Autodesk Inventor part; units mm, degrees
ref_plane "工作平面1" through (2.5, 0, 0) normal (1, 0, 0) x (0, 1, 0)
ref_plane "工作平面3" through (0, 0, 10) normal (0, 0, 1) x (1, 0, 0)
ref_plane "工作平面4" through (0, 0, -7) normal (0, 0, 1) x (1, 0, 0)
sketch "草图1" plane through (0, 0, 0) normal (1, 0, 0) x (0, 1, 0)
  circle A0 centre (0, 0) radius 10
  dimension "d0" = 20
extrude "拉伸1" add sketch "草图1" along normal blind 80
ref_plane "工作平面1" through (2.5, 0, 0) normal (1, 0, 0) x (0, 1, 0)
sketch "草图2" plane through (2.5, 0, 0) normal (1, 0, 0) x (0, 1, 0)
  circle A0 centre (0, 0) radius 10
  line L0 (6, -2.4628) -> (-6, -2.4628)
  line L1 (-6, -2.4628) -> (-6, 2.5372)
  line L2 (-6, 2.5372) -> (6, 2.5372)
  line L3 (6, 2.5372) -> (6, -2.4628)
  line L4 (6.59, 0.0372) -> (-6.5609, 0.0372)
  point P0 (10, 0)
  point P1 (-10, 0)
  dimension "d4" = 4
  dimension "d5" = 4
  dimension "d6" = 5
extrude "拉伸2" cut sketch "草图2" along normal blind 75 contours L0 L1 L4 L3 | L4 L1 L2 L3
ref_plane "工作平面3" through (0, 0, 10) normal (0, 0, 1) x (1, 0, 0)
sketch "草图5" plane through (0, 0, 10) normal (0, 0, 1) x (1, 0, 0)
  line L0 (-2.1953, 0) -> (98.9957, 0)
  line L1 (2.5, 6) -> (2.5, -6)
  line L2 (77.5, 6) -> (77.5, -6)
  line L3 (2.5, -6) -> (2.5, 6)
  line L4 (3.5, 4) -> (76.5, 4)
  line L5 (76.5, -4) -> (3.5, -4)
  line L6 (2.5, -3) -> (2.5, -2)
  arc A0 (3.5, 4) -> (3.5, 2) centre (3.5, 3) ccw
  arc A1 (3.5, -2) -> (3.5, -4) centre (3.5, -3) ccw
  line L7 (3.5, 2) -> (76.5, 2)
  line L8 (3.5, -2) -> (76.5, -2)
  arc A2 (76.5, 2) -> (76.5, 4) centre (76.5, 3) ccw
  circle A3 centre (76.5, -3) radius 1
  point P0 (0, 0)
  point P1 (3.5, 0)
  point P2 (76.5, 0)
  dimension "d52" = 8
  dimension "d53" = 1
  dimension "d54" = 1
  dimension "d55" = 1
extrude "拉伸3" cut sketch "草图5" against normal blind 7.5 contours A0 L4 A2 L7 | A1 L8 A3 L5
ref_plane "工作平面4" through (0, 0, -7) normal (0, 0, 1) x (1, 0, 0)
sketch "草图6" plane through (0, 0, -7) normal (0, 0, 1) x (1, 0, 0)
  line L0 (0, -10) -> (0, 10)
  line L1 (80, -10) -> (80, 10)
  line L2 (0, 1) -> (80, 1)
  line L3 (80, 1) -> (80, -1)
  line L4 (80, -1) -> (0, -1)
  line L5 (0, -1) -> (0, 1)
  line L6 (-22.5072, 0) -> (150.7978, 0)
  point P0 (0, 0)
  point P1 (0, -1)
  dimension "d39" = 2
extrude "拉伸4" add sketch "草图6" against normal blind 5.5
ref_plane "工作平面5" through (2.5, -6, -2.4628) normal (0, 0, 1) x (1, 0, 0)
sketch "草图7" plane through (2.5, -6, -2.4628) normal (0, 0, 1) x (1, 0, 0)
  point P0 (-2.5, 6)
properties part number "Inner_telescope_arm"
Could you check a few things on this model? Use its own coordinates, in mm. A direction names the side the tool comes from. Give positions to 0.01 mm unless a question says otherwise; leave off trailing zeros. Order: outer loops, then holes, each group sorted by start corner. A loop starts at its lowest first (then second) coordinate and runs counter-clockwise, first axis right, second up.
Item 1: I need wall thicknesses on line 1 (Z direction, x = 74, y = 0.25); line 2 (X direction, y = 5.5, z = 0.5); line 3 (Y direction, x = 19.5, z = 6.75). Which ranges of each line are inside material? Lowest first, please.
Item 2: If we section it at C-C, the plane y = 0: Write out the boundary of the cut face in (x, z), plus the area to 4 significant figures.
Item 3: I'm going to push flat-ended pins straight in: pin 1 (2.5 mm diameter, centred on x = 37, z = -1, fed in from +Y); pin 2 (5.5 mm diameter, centred on x = 50, z = 6, fed in from -Y); pin 3 (10 mm diameter, centred on x = 61, y = -6.5, fed in from -Z); pin 4 (6 mm diameter, centred on x = 30.5, z = 4.5, fed in from -Y). Where does each tip first touch, or does it pass through?
Item 4: For faces 5 (the face through (2.5, 3, 6.2)), 6 (the face through (39, 6, 0)), 7 (the face through (39, 0, -12.5)), which set-ups out of +Z, -Z, +X, -X, +Y, -Y let a thin tool reach every point of the face, with its end or its side?
Item 5: If we section it at A-A, the plane z = 0: Write out the boundary of the cut face in (x, y), plus the area to 3 significant figures.
Item 6: If we section it at D-D, the plane z = 3.75: Write out the boundary of the cut face in (x, y).
Item 7: If we section it at B-B, the plane x = 21: Write out the boundary of the cut face in (y, z).
Item 8: If we mould it in two halves opening along X, with no side actions, what happens to faces 1 (the face through (41, -1, -11)), 2 (the face through (77.5, 3, 6.2)), 3 (the face through (0, 0, -1)), 4 (the face through (80, 0, -1))? For each: pulls with the +X half, pulls with the -X half, needs draft (parallel to the pull), parting line crosses it, or undercut.
Values:
1. line 1: z = -12.5 to -2.46, 2.54 to 10
1. line 2: x = 0 to 2.5, 77.5 to 80
1. line 3: y = -7.38 to -4, -2 to 2, 4 to 7.38
2. outline: (0, -12.5) - (80, -12.5) - (80, 10) - (0, 10) - close; hole (2.5, -2.46) - (77.5, -2.46) - (77.5, 2.54) - (2.5, 2.54) - close
2. area: 1,425 mm2
3. pin 1: stops at y = 10
3. pin 2: stops at y = -9.46
3. pin 3: stops at z = -9.89
3. pin 4: stops at y = -9.89
4. face 5: +Z
4. face 6: none
4. face 7: -Z, +X, -X, +Y, -Y
5. outline: (0, -10) - (80, -10) - (80, 10) - (0, 10) - close; hole (2.5, -6) - (77.5, -6) - (77.5, 6) - (2.5, 6) - close
5. area: 700 mm2
6. outline: (0, -9.27) - (80, -9.27) - (80, 9.27) - (0, 9.27) - close; hole (3.5, -4) - (76.5, -4) arc R1 cw to (76.5, -2) - (3.5, -2) arc R1 ccw to start; hole (3.5, 2) - (76.5, 2) arc R1 ccw to (76.5, 4) - (3.5, 4) arc R1 ccw to start
7. outline: (-6, -2.46) - (-6, 2.54) - (-4, 2.54) - (-4, 9.17) arc R10 ccw to (-1, -9.95) - (-1, -12.5) - (1, -12.5) - (1, -9.95) arc R10 ccw to (4, 9.17) - (4, 2.54) - (6, 2.54) - (6, -2.46) - close; (-2, 2.54) - (2, 2.54) - (2, 9.8) arc R10 ccw to (-2, 9.8) - close
8. face 1: needs draft
8. face 2: undercut
8. face 3: pulls with the -X half
8. face 4: pulls with the +X half
